Here's how the part is built. I have some questions about the finished solid (model axes, mm). A direction names the side the tool comes from. Give positions to 0.01 mm unless a question says otherwise; leave off trailing zeros. Order: outer loops, then holes, each group sorted by start corner. A loop starts at its lowest first (then second) coordinate and runs counter-clockwise, first axis right, second up. Notation, with made-up numbers: (56, 37) -> (95, 37) arc R4 cw to (95, 41) -> close; hole circle Ø1 at (-35.5, 77). An arc over 180 degrees is marked (long way). Write each question's results on one line, items separated by ' | '. Start each with the question number.
Q1. For faces 1 (the face through (-9.18, -52.2, -0.03)), 2 (the face through (-25, 1, 0)), which set-ups out of +Z, -Z, +X, -X, +Y, -Y let a thin tool reach every point of the face, with its end or its side?
Q2. Imagine slicing it at B-B, the plane x = 17. Please give me the cut outline in (y, z), then the cut area to 3 significant figures.
Q3. Thinking about a two-plate mould opening in X: for faces 3 (the face through (9.23, -52.19, -0.03)), 4 (the face through (0, -73, 0)), 5 (the face through (0, 1, -10)), which applies, pulls with the +X half, pulls with the -X half, needs draft (parallel to the pull), parting line crosses it, or undercut?
Q4. Imagine slicing it at A-A, the plane z = -4.25. Please give me the cut outline in (x, y), then the cut area to 3 significant figures.
Q5. I need wall thicknesses on line 1 along Y through (x, z) = (-2, -5.5); line 2 along Y through (x, z) = (17.5, -4.5). Which ranges of each line are inside material? Lowest first, please. Write a range as [from, to].
Q6. I'm going to push flat-ended pins straight in: pin 1 (5 mm diameter, centred on x = -15.5, z = 3.5, fed in from -Y); pin 2 (1 mm diameter, centred on x = -11, z = -2, fed in from +Y); pin 3 (1 mm diameter, centred on x = 2, z = 4.5, fed in from -Y). Where does each tip first touch, or does it pass through?
Solid Edge part; units mm, degrees
sketch "Sketch1" plane through (0, 0, 0) normal (0, 0, 1) x (1, 0, 0)
  line L0 (25, -68.5857) -> (25, 68.5857)
  line L1 (-25, 68.5857) -> (-25, -68.5857)
  arc A0 (25, -68.5857) -> (-25, -68.5857) centre (0, 0) cw
  arc A1 (25, 68.5857) -> (-25, 68.5857) centre (0, 0) ccw
extrude "Protrusion1" add sketch "Sketch1" along normal mid plane 20
sketch "Sketch2" plane through (12.6763, -71.891, 0) normal (0.1736, -0.9848, 0) x (0, 0, -1)
  circle A0 centre (0, 0) radius 2
extrude "Wycięcie_1" cut sketch "Sketch2" against normal blind 20
mirror "Mirror1" about plane through (0, 0, 0) normal (1, 0, 0) of "Wycięcie_1"
mirror "Mirror2" about plane through (0, 0, 0) normal (0, -1, 0) of "Mirror1", "Wycięcie_1"
Geometry check:
1) face 1: none | face 2: +Z, -Z, -X, +Y, -Y
2) outline: (-70.99, -10) -> (70.99, -10) -> (70.99, 10) -> (-70.99, 10) -> close | area: 2,840 mm²
3) face 3: undercut | face 4: parting line crosses it | face 5: needs draft
4) outline: (-25, -68.59) arc R73 ccw to (25, -68.59) -> (25, 68.59) arc R73 ccw to (-25, 68.59) -> close | area: 7,150 mm²
5) line 1: [-72.97, 72.97] | line 2: [-70.87, 70.87]
6) pin 1: y = -71.83 | pin 2: y = 72.24 | pin 3: y = -72.98
